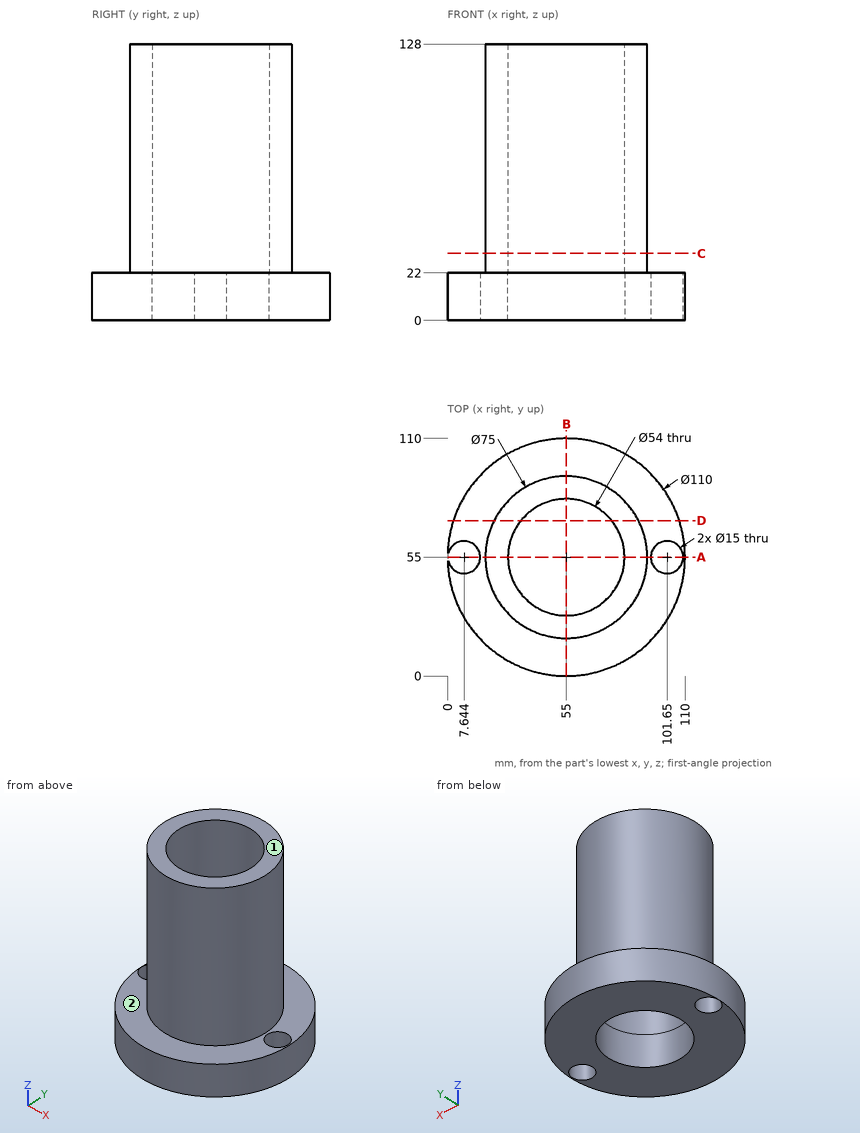
Answer from the drawing. Dimensions are ordinates in mm from the lowest x, y and z of the part. A direction names the side the tool comes from. Give positions to 0.01 mm unless a question says otherwise; leave off trailing zeros. Loops run counter-clockwise (first coordinate to the right, second up) from the corner with the lowest first, then second, coordinate; pieces in that order, holes last. Notation, with made-up numbers: (-3.75, 15) - (27.25, 15) arc R23 cw to (27.25, 35) - close; hole circle Ø7 at (22.25, 85). An arc over 180 degrees is marked (long way). Write each question's results on one line, items separated by ' | '.
1. Flat-ended cylindrical pins translate along their axes: P1, Ø10, axis at x = 71, z = 41.5, coming from the +Y side; P2, Ø12, axis at y = 77, z = 31.5, coming from the -X side (1 decimal); P3, Ø10, axis at x = 24.5, z = 74.5, coming from the -Y side (1 decimal); P4, Ø6, axis at x = 30.5, y = 33, coming from the -Z side. Find the tip coordinate at first contact, or state that the pin passes through.
Resolved:
P1: stops at y = 90.85 | P2: stops at x = 21.1 | P3: stops at y = 27.5 | P4: stops at z = 0
2. Find section C-C, the plane z = 31. Write down the section's boundary in (x, y), then the cut area to 3 significant figures.
Resolved:
outline: circle Ø75 at (55, 55); hole circle Ø54 at (55, 55) | area: 2,130 mm^2
3. Find section B-B, the plane x = 55. Write down the section's boundary in (y, z), then the cut area to 3 significant figures.
Resolved:
outline: (0, 0) - (28, 0) - (28, 128) - (17.5, 128) - (17.5, 22) - (0, 22) - close; (82, 0) - (110, 0) - (110, 22) - (92.5, 22) - (92.5, 128) - (82, 128) - close | area: 3,460 mm^2
4. Consider probe 1 along Y at (x, z) = (55, 15); probe 2 along X at (y, z) = (54.5, 61) (1 decimal); probe 3 along Z at (x, y) = (96, 81.5). Determine where each line is inside the solid, lowest interval first. Write a range as from..to.
Resolved:
probe 1: y = 0..28, 82..110 | probe 2: x = 17.5..28, 82..92.5 | probe 3: z = 0..22
5. Which of the six approach directions +Z, -Z, +X, -X, +Y, -Y give full straight-line access (tool end or side, diameter ignored) to the marked faces 1 and 2?
Resolved:
face 1: +Z, +X, -X, +Y, -Y | face 2: +Z
6. Find section D-D, the plane y = 72. Write down the section's boundary in (x, z) (1 decimal).
Resolved:
outline: (2.7, 0) - (34, 0) - (34, 128) - (21.6, 128) - (21.6, 22) - (2.7, 22) - close; (76, 0) - (107.3, 0) - (107.3, 22) - (88.4, 22) - (88.4, 128) - (76, 128) - close
7. Find section A-A, the plane y = 55. Write down the section's boundary in (x, z), then the cut area to 3 significant figures.
Resolved:
outline: (0, 0) - (0.14, 0) - (0.14, 22) - (0, 22) - close; (15.14, 0) - (28, 0) - (28, 128) - (17.5, 128) - (17.5, 22) - (15.14, 22) - close; (82, 0) - (94.15, 0) - (94.15, 22) - (92.5, 22) - (92.5, 128) - (82, 128) - close; (109.15, 0) - (110, 0) - (110, 22) - (109.15, 22) - close | area: 2,800 mm^2
